Could you check a few things on this model? Use its own coordinates, in mm. A direction names the side the tool comes from. Coordinates: 2 decimals unless noted, no trailing zeros. Write each loop counter-clockwise with the first axis right and the second up, starting at its lowest first coordinate (ties: lowest second). Pieces come first, ordered by that corner, then holes. Notation, with made-up numbers: (29, 35.5) - (62, 35.5) arc R22 cw to (62, 43.5) - close; hole circle Ø7 at (56.5, 43). An arc over 180 degrees is marked (long way). Write item = value, one per line. Start each with the question number.
```python
from build123d import *

# Parameters (mm, degrees)
SKETCH2_R           = 9.525
BOSS_EXTRUDE1_DEPTH = 63.5
SKETCH3_W           = 19.05
SKETCH3_H           = 25.4
BOSS_EXTRUDE2_DEPTH = 50.8
SKETCH4_W           = 25.4
SKETCH4_H           = 19.05
BOSS_EXTRUDE3_DEPTH = 25.4
SKETCH5_2_R         = 9.525
BOSS_EXTRUDE4_DEPTH = 127
BOSS_EXTRUDE4_TAPER = 1.5
SKETCH8_W           = 19.05
SKETCH8_H           = 63.5
BOSS_EXTRUDE5_DEPTH = 12.7
SKETCH9_W           = 19.05
SKETCH9_H           = 12.7
BOSS_EXTRUDE6_DEPTH = 25.4
FILLET2_R           = 9.525
SKETCH12_R          = 4.7625
CUT_EXTRUDE1_DEPTH  = 206.928278116
FILLET3_R           = 9.525


with BuildPart() as part:
    # Sketch2 → Boss-Extrude1 (new body)
    with BuildSketch(Plane.XY):
        Circle(SKETCH2_R)
    extrude(amount=BOSS_EXTRUDE1_DEPTH)

    # Sketch3 → Boss-Extrude2 (add)
    with BuildSketch(Plane(origin=(0, 0, 0), x_dir=(1, 0, 0), z_dir=(0, 1, 0))):
        with Locations((0, -31.75)):
            Rectangle(SKETCH3_W, SKETCH3_H)
    extrude(amount=-BOSS_EXTRUDE2_DEPTH)

    # Sketch4 → Boss-Extrude3 (add)
    with BuildSketch(Plane(origin=(0, 0, 0), x_dir=(0, 0, -1), z_dir=(0.8660254037844398, 0.499999999999998, 0))):
        with Locations((-31.75, 0)):
            Rectangle(SKETCH4_W, SKETCH4_H)
    extrude(amount=BOSS_EXTRUDE3_DEPTH)

    # Sketch6 → Loft1 section 0
    with BuildSketch(Plane(origin=(21.997045256, 12.7, 0), x_dir=(0, 0, -1), z_dir=(0.8660254037844397, 0.4999999999999981, 0))):
        with BuildLine():
            Line((-44.45, 9.525), (-44.45, -9.525))
            Line((-44.45, -9.525), (-19.05, -9.525))
            Line((-19.05, -9.525), (-19.05, 9.525))
            Line((-19.05, 9.525), (-44.45, 9.525))
        make_face()
    # Sketch5 for Loft1 → Loft1 section 1
    with BuildSketch(Plane(origin=(54.99261314, 31.75, 0), x_dir=(0, 0, -1), z_dir=(0.8660254037844397, 0.4999999999999981, 0))):
        with BuildLine():
            # circular arc as an exact rational Bezier (weights 1, cos(half-angle), 1)
            Bezier((-39.37, 5.715), (-43.65625, 0), (-39.37, -5.715), weights=[1, 0.8, 1])
            Bezier((-39.37, -5.715), (-31.75, -15.875), (-24.13, -5.715), weights=[1, 0.6, 1])
            Bezier((-24.13, -5.715), (-19.84375, 0), (-24.13, 5.715), weights=[1, 0.8, 1])
            Bezier((-24.13, 5.715), (-31.75, 15.875), (-39.37, 5.715), weights=[1, 0.6, 1])
        make_face()
    loft()

    # Sketch5<2> → Boss-Extrude4 (add)
    with BuildSketch(Plane(origin=(54.99261314, 31.75, 0), x_dir=(0, 0, -1), z_dir=(0.8660254037844397, 0.4999999999999981, 0))):
        with Locations((-31.75, 0)):
            Circle(SKETCH5_2_R)
    extrude(amount=BOSS_EXTRUDE4_DEPTH, taper=BOSS_EXTRUDE4_TAPER)

    # Sketch8 → Boss-Extrude5 (add)
    with BuildSketch(Plane.XZ.offset(50.8)):
        with Locations((0, 31.75)):
            Rectangle(SKETCH8_W, SKETCH8_H)
    extrude(amount=BOSS_EXTRUDE5_DEPTH)

    # Sketch9 → Boss-Extrude6 (add)
    with BuildSketch(Plane.XZ.offset(63.5)):
        with Locations((0, 57.15)):
            Rectangle(SKETCH9_W, SKETCH9_H)
        with Locations((0, 6.35)):
            Rectangle(SKETCH9_W, SKETCH9_H)
    extrude(amount=BOSS_EXTRUDE6_DEPTH)

    # Fillet2
    fillet2_edges = [part.edges().sort_by_distance(p)[0] for p in [
        (9.525, -88.9, 6.35),
        (9.525, -88.9, 57.15),
        (-9.525, -88.9, 57.15),
        (-9.525, -88.9, 6.35),
    ]]
    fillet(fillet2_edges, radius=FILLET2_R - 0.0001)  # a hair under: the kernel refuses the full size

    # Sketch12 → Cut-Extrude1 (cut, through all)
    with BuildSketch(Plane(origin=(0, 0, 0), x_dir=(-1, 0, 0), z_dir=(0, 0, -1))):
        with Locations((0, -79.375)):
            Circle(SKETCH12_R)
    extrude(amount=-CUT_EXTRUDE1_DEPTH, mode=Mode.SUBTRACT)

    # Fillet3
    fillet3_edges = [part.edges().sort_by_distance(p)[0] for p in [
        (0, -50.8, 0),
        (0, -50.8, 63.5),
    ]]
    fillet(fillet3_edges, radius=FILLET3_R)


solid = part.part
```
1) Which directions (+Z, -Z, +X, -X, +Y, -Y) give clear straight access to the entire face, cutting with the end or side of a thin tool? Please do faces 1 (the cylindrical face through (-6.809, -86.036, 57.239)), 2 (the cylindrical face through (0.13, -53.66, 60.78)), 3 (the cylindrical face through (-9.516, 0.419, 31.306)), 4 (the flat face through (0, -63.5, 32)), 5 (the flat face through (0, -50.8, 14)).
2) If I drill on probe 1 along Y at (x, z) = (0, 58.75) (1 decimal); probe 2 along Y at (x, z) = (0, 56) (1 decimal); probe 3 along X at (y, z) = (-56.5, 37) (3 decimals), over which ranges is the centre line in solid material (lowest first)? Write a range as [from, to].
3) Suppose I cut it at A-A on y = -44.5. Please give me the cut outline in (x, z) (3 decimals).
4) For P1, Ø5, axis at x = -2.5, z = 16.5, coming from the +Y side (3 decimals); P2, Ø8.5, axis at x = 0, y = -79.375, coming from the -Z side; P3, Ø3, axis at y = -16, z = 20.5, coming from the +X side (3 decimals); P4, Ø15, axis at x = 0, z = 26, coming from the -Y side, each with a flat end and sliding along its axis, tell me the tip position at first contact or that it passes through.
5) Thinking about a two-plate mould opening in Z: for faces 6 (the conical face through (113.14, 59.81, 37.97)), 7 (the flat face through (4, -22, 19.05)), 8 (the flat face through (-9.525, -48, 31)), 9 (the flat face through (0, -73, 50.8)), which applies, +Z half, -Z half, draft (parallel to the pull), parting line (faces both ways), or undercut?
Reply:
q1.face_1 = +Z, -Z, -X, -Y
q1.face_2 = +Z, +X, -X
q1.face_3 = none
q1.face_4 = +X, -X, -Y
q1.face_5 = -Z, +X, -X
q2.probe_1 = [-88.9, -84.1], [-74.6, -52.1], [-9.5, 9.5]
q2.probe_2 = [-88.9, -84.1], [-74.6, -51], [-9.5, 9.5]
q2.probe_3 = [-9.525, 9.525]
q3.outline = (-9.525, 19.05) - (9.525, 19.05) - (9.525, 44.45) - (-9.525, 44.45) - close
q4.P1 = 9.525
q4.P2 = through
q4.P3 = 9.525
q4.P4 = -63.5
q5.face_6 = parting line
q5.face_7 = -Z half
q5.face_8 = draft
q5.face_9 = undercut
